Input: part model. Units: mm. Frame: model coordinates. A direction names the side the tool comes from. Round coordinates to 2 decimals unless told otherwise and drop trailing zeros. Order: outer loops, then holes, each group sorted by start corner. A loop starts at its lowest first (then second) coordinate and runs counter-clockwise, first axis right, second up.
Item 1: Cut plane A-A on z = -404. Output: boundary loops of the cut face in (x, y).
Item 2: Mould query, pull axis X, two halves, no side actions, for faces 4 (the flat face through (-1, -10, -331)), 5 (the flat face through (0, -12, 7)), 6 (the cylindrical face through (79, 0, 31)). Classes: released by +X, released by -X, zero draft, split by the parting line, or undercut.
Item 3: Line query: L1, parallel to Z at x = -49, y = 16; L2, parallel to Z at x = 66.5, y = 16; L3, parallel to Y at x = 6.5, z = -227. Output: solid intervals per line, ascending.
Item 4: Reachability of faces 1 (the flat face through (-1, 10, 35)), 2 (the flat face through (-31.91, -5.92, 6.71)), 3 (the flat face through (-1, 10, -331)) from +Z, -Z, +X, -X, +Y, -Y: full face, straight path, thin tool, end or side. Return the list, or none.
Item 5: First-contact query: pin 1 (8 mm diameter, centred on x = 10, z = -362, fed in from +Y); pin 2 (4 mm diameter, centred on x = 61, y = -10.5, fed in from +Z); pin 3 (12 mm diameter, centred on x = -3, z = 10, fed in from -Y). Flat tips, straight axial feed; report the tip coordinate or a pass-through.
```python
from build123d import *

# Parameters (mm, degrees)
EXTRUDE_1_DEPTH      = 18
CHAMFER_1_SIZE       = 5
CHAMFER_2_SIZE       = 5
CUT_EXTRUDE_1_DEPTH  = 8
EXTRUDE_2_REACH      = 696.741
EXTRUDE_2_END_RADIUS = 240


with BuildPart() as part:
    # Sketch 4 → Loft 1 section 0
    with BuildSketch(Plane(origin=(0, 10, 0), x_dir=(1, 0, 0), z_dir=(0, 1, 0))):
        with BuildLine():
            Line((25, 0), (-25, 0))
            Line((-25, 0), (-25, 630))
            Line((-25, 630), (0, 672.857142857))
            Line((0, 672.857142857), (25, 630))
            Line((25, 630), (25, 0))
        make_face()
    # Sketch 1 → Loft 1 section 1
    with BuildSketch(Plane(origin=(0, 0, 0), x_dir=(1, 0, 0), z_dir=(0, 1, 0))):
        with BuildLine():
            Line((-35, 0), (35, 0))
            Line((35, 0), (35, 630))
            Line((35, 630), (0, 690))
            Line((0, 690), (-35, 630))
            Line((-35, 630), (-35, 0))
        make_face()
    loft_1 = loft()

    # Mirror 1: Loft 1 across plane
    add(loft_1.mirror(Plane.ZX))



with BuildPart() as body_2:
    # Sketch 5 → Extrude 1 (new, symmetric)
    with BuildSketch(Plane(origin=(0, 0, 0), x_dir=(1, 0, 0), z_dir=(0, 1, 0))):
        with BuildLine():
            ThreePointArc((-66.346774613, -65.189169183), (0, -55.5), (66.346774613, -65.189169183))
            ThreePointArc((66.346774613, -65.189169183), (73.061224406, -64.270510235), (76.791165228, -58.612302768))
            ThreePointArc((76.791165228, -58.612302768), (79, -30.5), (76.791165228, -2.387697232))
            ThreePointArc((76.791165228, -2.387697232), (0, -15.004503167), (-76.791165228, -2.387697232))
            ThreePointArc((-76.791165228, -2.387697232), (-79, -30.5), (-76.791165228, -58.612302768))
            ThreePointArc((-76.791165228, -58.612302768), (-73.061224406, -64.270510235), (-66.346774613, -65.189169183))
        make_face()
    extrude(amount=EXTRUDE_1_DEPTH, both=True)

    # Chamfer 1
    chamfer_1_edges = [body_2.edges().sort_by_distance(p)[0] for p in [
        (0, 18, 15.004503167),
        (-79, 18, 30.5),
        (-73.061224406, 18, 64.270510235),
        (0, 18, 55.5),
        (73.061224406, 18, 64.270510235),
        (0, -18, 55.5),
        (-73.061224406, -18, 64.270510235),
        (-79, -18, 30.5),
        (79, -18, 30.5),
        (73.061224406, -18, 64.270510235),
        (79, 18, 30.5),
    ]]
    chamfer(chamfer_1_edges, length=CHAMFER_1_SIZE)

    # Chamfer 2
    chamfer_2_edges = [body_2.edges().sort_by_distance(p)[0] for p in [
        (0, -18, 15.004503167),
    ]]
    chamfer(chamfer_2_edges, length=CHAMFER_2_SIZE)

    # Sketch 6 → Cut-Extrude 1 (cut)
    with BuildSketch(Plane(origin=(0, 18, 0), x_dir=(1, 0, 0), z_dir=(0, 1, 0))):
        with BuildLine():
            ThreePointArc((67.221840199, -55.023712607), (68.932610365, -35.286223394), (68.335500378, -15.483731767))
            ThreePointArc((68.335500378, -15.483731767), (0, -25.004503167), (-68.335500378, -15.483731767))
            ThreePointArc((-68.335500378, -15.483731767), (-68.932610365, -35.286223394), (-67.221840199, -55.023712607))
            ThreePointArc((-67.221840199, -55.023712607), (0, -45.5), (67.221840199, -55.023712607))
        make_face()
    cut_extrude_1 = extrude(amount=-CUT_EXTRUDE_1_DEPTH, mode=Mode.SUBTRACT)

    # Mirror 2: Cut-Extrude 1 across plane
    add(cut_extrude_1.mirror(Plane.ZX), mode=Mode.SUBTRACT)


with BuildPart() as part_1:
    add(part.part)

    add(body_2.part)  # Extrude 2 merges body 2
    # Extrude 2: up to this cylinder (the profile starts inside it)
    extrude_2_end = Plane(origin=(0, 0, -224.995496833), z_dir=(0, -1, 0)) * Cylinder(EXTRUDE_2_END_RADIUS, 1874.482, mode=Mode.PRIVATE)
    # Sketch 7 → Extrude 2 (add, up to the surface)
    with BuildSketch(Plane.XY, mode=Mode.PRIVATE) as extrude_2_sk1:
        Polygon((-25.828427125, 12), (-37.828427125, 0), (-25.828427125, -12), (25.828427125, -12), (37.828427125, 0), (25.828427125, 12), align=None)
    extrude_2_tool1 = extrude(extrude_2_sk1.sketch, amount=EXTRUDE_2_REACH, mode=Mode.PRIVATE) & extrude_2_end
    add(extrude_2_tool1.solids().sort_by_distance((0, 0, 0))[0])


solid = part_1.part
```
From the geometry:
1. outline: (-35, 0) - (-25, -10) - (25, -10) - (35, 0) - (25, 10) - (-25, 10) - close
2. face 4: zero draft
2. face 5: undercut
2. face 6: released by +X
3. L1: z = 13.01 to 20.16, 50.51 to 57.67
3. L2: z = 8.73 to 16, 54.82 to 62.11
3. L3: y = -10 to 10
4. face 1: +Y
4. face 2: -Z, -Y
4. face 3: -Z, +X, -X, +Y
5. pin 1: stops at y = 10
5. pin 2: stops at z = 64.22
5. pin 3: stops at y = -14.01
